Design review of the part built by this model. Coordinates are the model's own, in mm. Give positions to 0.01 mm unless a question says otherwise; leave off trailing zeros. Loops run counter-clockwise (first coordinate to the right, second up) from the corner with the lowest first, then second, coordinate; pieces in that order, holes last. Notation, with made-up numbers: M 73.5,6.25 L 96.5,6.25 A22 ccw 96.5,32.25 Z; hole C 71,69 d2. An arc over 180 degrees is marked long. Use CSV: the item, a comma, the result in double quotes.
from build123d import *

# Parameters (mm, degrees)
SKETCH_1_W               = 195
SKETCH_1_H               = 10
EXTRUDE_1_DEPTH          = 1.5
CUT_EXTRUDE_1_DEPTH      = 12
CUT_EXTRUDE_1_DEPTH_BACK = 15
SKETCH_2_R               = 1
CUT_EXTRUDE_2_DEPTH      = 32
CUT_EXTRUDE_2_DEPTH_BACK = 31
SKETCH_3_R               = 1.5
SKETCH_3_R_2             = 1
SKETCH_4_W               = 17
SKETCH_4_H               = 3
SKETCH_4_W_2             = 25
SKETCH_4_W_3             = 15
CUT_EXTRUDE_3_DEPTH      = 10


with BuildPart() as part:
    # Sketch 1 → Extrude 1 (new body)
    with BuildSketch(Plane.XY):
        with Locations((-102.5, -5)):
            Rectangle(SKETCH_1_W, SKETCH_1_H)
    extrude(amount=EXTRUDE_1_DEPTH)

    # Sketch 2 → Cut-Extrude 1 (cut, two sides: drawn at the far end of the back side and taken through both)
    with BuildSketch(Plane.XY.offset(1.5).offset(-CUT_EXTRUDE_1_DEPTH_BACK)):
        with Locations((-192, -5)):
            Circle(SKETCH_2_R)
    extrude(amount=CUT_EXTRUDE_1_DEPTH + CUT_EXTRUDE_1_DEPTH_BACK, mode=Mode.SUBTRACT)

    # Sketch 3 → Cut-Extrude 2 (cut, two sides: drawn at the far end of the back side and taken through both)
    with BuildSketch(Plane.XY.offset(1.5).offset(-CUT_EXTRUDE_2_DEPTH_BACK)):
        with Locations((-13, -5)):
            Circle(SKETCH_3_R)
        with Locations((-8, -5)):
            Circle(SKETCH_3_R_2)
        with Locations((-18, -5)):
            Circle(SKETCH_3_R_2)
    extrude(amount=CUT_EXTRUDE_2_DEPTH + CUT_EXTRUDE_2_DEPTH_BACK, mode=Mode.SUBTRACT)

    # Sketch 4 → Cut-Extrude 3 (cut)
    with BuildSketch(Plane(origin=(0, 0, 0), x_dir=(-1, 0, 0), z_dir=(0, 0, -1))):
        with Locations((95.5, -7.5)):
            Rectangle(SKETCH_4_W, SKETCH_4_H)
        with Locations((151.5, -7.5)):
            Rectangle(SKETCH_4_W_2, SKETCH_4_H)
        with Locations((49.5, -7.5)):
            Rectangle(SKETCH_4_W_3, SKETCH_4_H)
    extrude(amount=-CUT_EXTRUDE_3_DEPTH, mode=Mode.SUBTRACT)


solid = part.part
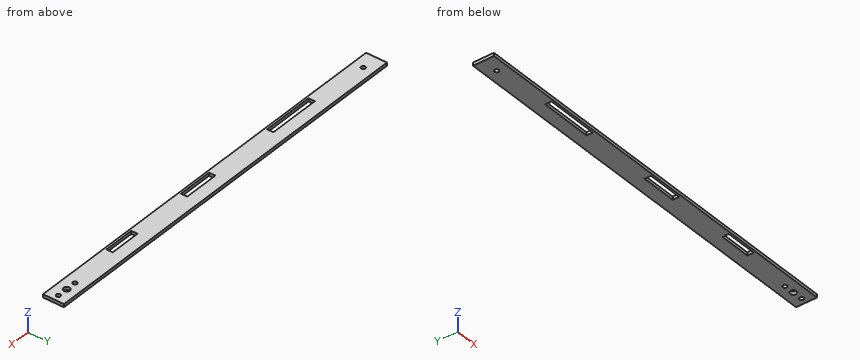
(1) Clearance check with a flat-ended pin moving along its axis: P1, Ø1.6, axis at x = -192, y = -5, coming from the +Z side. State where the tip first meets the part, or that it passes through.
A:
P1,"through"
(2) We need section B-B on x = -146. State the section outline as (y, z) points.
A:
outline,"M -10,0 L -9,0 L -9,1.5 L -10,1.5 Z; M -6,0 L 0,0 L 0,1.5 L -6,1.5 Z"
(3) We need section A-A on z = 0.7. State the section outline as (x, y) points, then the cut area to 3 significant figures.
A:
outline,"M -200,-10 L -5,-10 L -5,0 L -200,0 Z; hole C -192,-5 d2; hole M -164,-9 L -139,-9 L -139,-6 L -164,-6 Z; hole M -104,-9 L -87,-9 L -87,-6 L -104,-6 Z; hole M -57,-9 L -42,-9 L -42,-6 L -57,-6 Z; hole C -18,-5 d2; hole C -13,-5 d3; hole C -8,-5 d2"
area,"1,760 mm²"
(4) Wall thickness on line 1 along X through (y, z) = (-8.5, 0.8); line 2 along X through (y, z) = (-5, 0.5); line 3 along Y through (x, z) = (-8, 0.4): over which ranges is each line inside the solid? List them lowest first. Write a range as [from, to].
A:
line 1,"[-200, -164], [-139, -104], [-87, -57], [-42, -5]"
line 2,"[-200, -193], [-191, -19], [-17, -14.5], [-11.5, -9], [-7, -5]"
line 3,"[-10, -6], [-4, 0]"
